Check sheet for the modelled part. Datum: model origin and axes. Units: mm. A direction names the side the tool comes from. Round coordinates to 2 decimals unless told otherwise and drop trailing zeros. Order: outer loops, then holes, each group sorted by start corner. A loop starts at its lowest first (then second) coordinate and runs counter-clockwise, first axis right, second up. Notation, with made-up numbers: (-35.5, 57) -> (-17.5, 57) arc R12 cw to (-17.5, 77) -> close; hole circle Ø8 at (-34, 58.5). An arc over 180 degrees is marked (long way). Answer as CSV lines item,"result". Start each with the question number.
from build123d import *

# Parameters (mm, degrees)
F1_DEPTH = 50
F3_DEPTH = 50
F5_DEPTH = 50
F6_W     = 54.105216
F6_H     = 17.56295
F6_R     = 19.170726
F6_W_2   = 15.580038
F6_H_2   = 14.446942
F7_DEPTH = 25


with BuildPart() as f1:
    # F0 (on Top) → F1 (new body)
    with BuildSketch(Plane.XY):
        Polygon((-38.042759, 65.710473), (-75.928318, -0.090759), (-37.88556, -65.801232), (38.042759, -65.710473), (75.928318, 0.090759), (37.88556, 65.801232), align=None)
    extrude(amount=F1_DEPTH)

    # F2 (on face) → F3 (join)
    with BuildSketch(Plane.XY.offset(50)):
        Polygon((-34.905945, 60.566627), (-69.90521, 0.053879), (-34.999265, -60.512748), (34.905945, -60.566627), (69.90521, -0.053879), (34.999265, 60.512748), align=None)
    extrude(amount=F3_DEPTH)

    # F4 (on face) → F5 (join)
    with BuildSketch(Plane.XY.offset(100)):
        Polygon((-31.442505, 54.790029), (-63.170809, 0.165007), (-31.728305, -54.625022), (31.442505, -54.790029), (63.170809, -0.165007), (31.728305, 54.625022), align=None)
    extrude(amount=F5_DEPTH)

    # F6 (on face) → F7 (join)
    with BuildSketch(Plane.XY.offset(150)):
        with Locations((2.124549, 35.409174)):
            Rectangle(F6_W, F6_H)
        with Locations((-31.160073, -3.399281)):
            Circle(F6_R)
        with Locations((27.619156, 7.223471)):
            Rectangle(F6_W_2, F6_H_2)
        Polygon((2.832735, -24.521915), (2.832735, -32.699312), (9.914569, -36.78801), (16.996402, -32.699312), (16.996402, -24.521915), (9.914569, -20.433216), align=None)
    extrude(amount=F7_DEPTH)


solid = f1.part
1) Section check C-C on y = 20.5. Record the cut outline in (x, z).
2) Section check B-B on x = 59. Record the cut outline in (y, z), then the cut area to 3 significant figures.
3) Material ranges on line 1 along Z through (x, y) = (-47, -35.5); line 2 along Y through (x, z) = (24, 159); line 3 along Z through (x, y) = (-39.5, -24.5), recorded low to high.
4) Mould release check, pull along X, two halves, no side actions. Record for faces 6 (the face through (13.51, -22.51, 162.32)), 7 (the face through (19.829, 7, 162)), 8 (the face through (2, 44.191, 162)): released by +X, released by -X, zero draft, split by the parting line, or undercut.
5) Access from +Z, -Z, +X, -X, +Y, -Y to the whole of each face (thin tool, end or side, straight path). Record for faces 1 (the face through (-33.656, 15.608, 162.325)), 2 (the face through (47.085, -27.86, 124.65)), 3 (the face through (-52.7, -29.8, 74.6)), 4 (the face through (-24.928, 35, 162)), 5 (the face through (52.7, 29.8, 74.6)).
6) Section check D-D on z = 108. Record the cut outline in (x, y) (1 decimal).
7) Depth check by flat-ended pin: pin 1 Ø5 at (x, y) = (-45.5, 10) entering from -Z; pin 2 Ø1.5 at (y, z) = (-24, 42.5) entering from -X; pin 3 Ø8 at (x, z) = (29, 159.5) entering from -Y; pin 4 Ø6.5 at (y, z) = (-30, 165.5) entering from -X. Enter the tip coordinate at first touch or a pass-through.
8) Section check A-A on z = 162.5. Record the cut outline in (x, y), then the cut area to 3 significant figures.
Solutions:
1,outline,"(-64.07, 0) -> (64.11, 0) -> (64.11, 50) -> (58.06, 50) -> (58.06, 100) -> (51.31, 100) -> (51.31, 150) -> (-51.36, 150) -> (-51.36, 100) -> (-58.08, 100) -> (-58.08, 50) -> (-64.07, 50) -> close"
2,outline,"(-29.31, 0) -> (29.33, 0) -> (29.33, 50) -> (18.87, 50) -> (18.87, 100) -> (7.1, 100) -> (7.1, 150) -> (-7.35, 150) -> (-7.35, 100) -> (-18.91, 100) -> (-18.91, 50) -> (-29.31, 50) -> close"
2,area,"5,540 mm^2"
3,line 1,"z = 0 to 100"
3,line 2,"y = 0 to 14.45, 26.63 to 44.19"
3,line 3,"z = 0 to 150"
4,face 6,"released by +X"
4,face 7,"undercut"
4,face 8,"zero draft"
5,face 1,"+Z"
5,face 2,"+Z, +X, -Y"
5,face 3,"+Z, -X, -Y"
5,face 4,"+Z, -X, +Y"
5,face 5,"+Z, +X, +Y"
6,outline,"(-63.2, 0.2) -> (-31.7, -54.6) -> (31.4, -54.8) -> (63.2, -0.2) -> (31.7, 54.6) -> (-31.4, 54.8) -> close"
7,pin 1,"stops at z = 0"
7,pin 2,"stops at x = -62.52"
7,pin 3,"stops at y = 0"
7,pin 4,"stops at x = 2.83"
8,outline,"circle Ø38.34 at (-31.16, -3.4); (-24.93, 26.63) -> (29.18, 26.63) -> (29.18, 44.19) -> (-24.93, 44.19) -> close; (2.83, -32.7) -> (9.91, -36.79) -> (17, -32.7) -> (17, -24.52) -> (9.91, -20.43) -> (2.83, -24.52) -> close; (19.83, 0) -> (35.41, 0) -> (35.41, 14.45) -> (19.83, 14.45) -> close"
8,area,"2,500 mm^2"
